Part model, mm, in its own coordinate system. Face numbers are marked on the shaded views. A direction names the side the tool comes from. Give positions to 0.01 mm unless a question says otherwise; leave off trailing zeros. Write each loop counter-clockwise with the first axis right and the second up, starting at its lowest first coordinate (ties: lowest second). Pieces come first, ordered by that corner, then holes. Notation, with made-up numbers: (12.5, 63) - (36.5, 63) arc R19 cw to (36.5, 81) - close; hole circle Ø2 at (40.5, 20.25). An arc over 180 degrees is marked (long way). Answer as a JSON object with one key per item and string values. Group by question number.
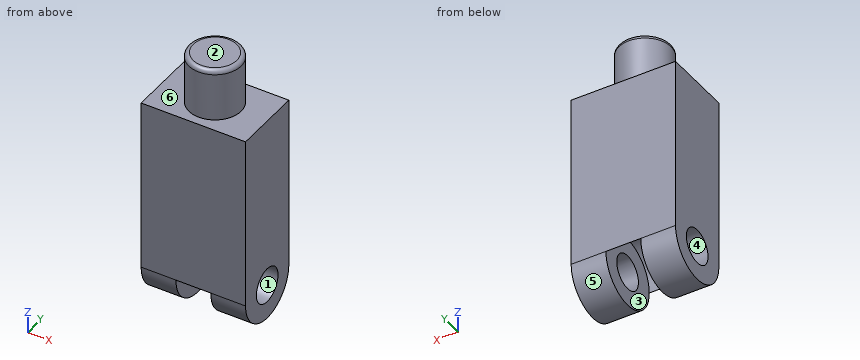
```python
from build123d import *

# Parameters (mm, degrees)
SKETCH_1_W               = 60
SKETCH_1_H               = 40
EXTRUDE_1_DEPTH          = 100
SKETCH_6_R               = 20
EXTRUDE_2_DEPTH          = 20
EXTRUDE_START            = -20
SKETCH_7_R               = 20
EXTRUDE_3_DEPTH          = 20
CUT_EXTRUDE_1_DEPTH      = 120.268604419
CUT_EXTRUDE_1_DEPTH_BACK = 120.268604419
SKETCH_8_R               = 10
SKETCH_9_R               = 20
CUT_EXTRUDE_2_DEPTH      = 20
SKETCH_10_R              = 15
EXTRUDE_4_DEPTH          = 30
FILLET_1_R               = 2.5


with BuildPart() as part:
    # 스케치1 → 보스-돌출1 (new body)
    with BuildSketch(Plane.XY):
        with Locations((20, 5)):
            Rectangle(SKETCH_1_W, SKETCH_1_H)
    extrude(amount=EXTRUDE_1_DEPTH)

    # 스케치6 → 보스-돌출2 (add)
    with BuildSketch(Plane(origin=(50, 0, 0), x_dir=(0, 0, -1), z_dir=(1, 0, 0))):
        with Locations((0, 5)):
            Circle(SKETCH_6_R)
    extrude(amount=-EXTRUDE_2_DEPTH)

    # 스케치7 → 보스-돌출3 (add)
    with BuildSketch(Plane.ZY.offset(10).offset(EXTRUDE_START)):
        with Locations((0, 5)):
            Circle(SKETCH_7_R)
    extrude(amount=EXTRUDE_3_DEPTH)

    # 스케치8 → 컷-돌출1 (cut, two sides: drawn at the far end of the back side and taken through both)
    with BuildSketch(Plane.ZY.offset(10).offset(-CUT_EXTRUDE_1_DEPTH_BACK)):
        with Locations((0, 5)):
            Circle(SKETCH_8_R)
    extrude(amount=CUT_EXTRUDE_1_DEPTH + CUT_EXTRUDE_1_DEPTH_BACK, mode=Mode.SUBTRACT)

    # 스케치9 → 컷-돌출2 (cut)
    with BuildSketch(Plane.ZY.offset(-30)):
        with Locations((0, 5)):
            Circle(SKETCH_9_R)
    extrude(amount=CUT_EXTRUDE_2_DEPTH, mode=Mode.SUBTRACT)

    # 스케치10 → 보스-돌출4 (add)
    with BuildSketch(Plane.XY.offset(100)):
        with Locations((20, 5)):
            Circle(SKETCH_10_R)
    extrude(amount=EXTRUDE_4_DEPTH)

    # 필렛1
    fillet_1_edges = [part.edges().sort_by_distance(p)[0] for p in [
        (5, 5, 130),
    ]]
    fillet(fillet_1_edges, radius=FILLET_1_R)


solid = part.part
```
1) Saw through at C-C (x = -6). List the corners of the cut face in (y, z).
2) Saw through at B-B (z = 8). List the corners of the cut face in (x, y), and give its area (3 significant figures).
3) Which spindle directions (+Z, -Z, +X, -X, +Y, -Y) get a long thin tool onto all of the face, cutting with end or side? Do the marked faces 5 and 6. Say none if no direction does.
4) Saw through at D-D (x = 20). List the corners of the cut face in (y, z), and give its area (3 significant figures).
5) Drop flat-ended pins along their axis: P1, Ø12, axis at y = 5, z = 0, coming from the -X side; P2, Ø1.5, axis at x = -1, y = 13.5, coming from the -Z side; P3, Ø10, axis at x = 36, y = 20.5, coming from the -Z side; P4, Ø6, axis at x = 24.5, y = -7, coming from the -Z side. Give the stop position or say it passes through.
6) Two-plate mould, pull along Z, no slides. Class the marked faces 1, 2, 3 and 4: +Z half, -Z half, draft (parallel to the pull), parting line (faces both ways), or undercut.
7) Saw through at A-A (y = 5). List the corners of the cut face in (x, z).
8) Drill centre lines: line 1 along Z through (x, y) = (4, 5); line 2 along Y through (x, z) = (42.5, 0); line 3 along Z through (x, y) = (7, 14). Where is each one in solid material? Low to high. Write a range as from..to.
Checks:
{
 "1": {"outline": "(-15, 0) arc R20 ccw to (25, 0) - (25, 100) - (-15, 100) - close; hole circle Ø20 at (5, 0)"},
 "2": {"outline": "(-10, -15) - (50, -15) - (50, -1) - (30, -1) - (30, -13.33) - (10, -13.33) - (10, -1) - (-10, -1) - close; (-10, 11) - (10, 11) - (10, 23.33) - (30, 23.33) - (30, 11) - (50, 11) - (50, 25) - (-10, 25) - close", "area": "1,190 mm2"},
 "3": {"face 5": "-Z, +X, -X", "face 6": "+Z"},
 "4": {"outline": "(-15, 0) arc R20 cw to (25, 0) - (25, 100) - (20, 100) - (20, 127.5) arc R2.5 ccw to (17.5, 130) - (-7.5, 130) arc R2.5 ccw to (-10, 127.5) - (-10, 100) - (-15, 100) - close", "area": "4,270 mm2"},
 "5": {"P1": "through", "P2": "z = -18.44", "P3": "z = -17.02", "P4": "z = 13.23"},
 "6": {"face 1": "undercut", "face 2": "+Z half", "face 3": "draft", "face 4": "undercut"},
 "7": {"outline": "(-10, -20) - (10, -20) - (10, -10) - (-10, -10) - close; (-10, 10) - (10, 10) - (10, 20) - (30, 20) - (30, 10) - (50, 10) - (50, 100) - (35, 100) - (35, 127.5) arc R2.5 ccw to (32.5, 130) - (7.5, 130) arc R2.5 ccw to (5, 127.5) - (5, 100) - (-10, 100) - close; (30, -20) - (50, -20) - (50, -10) - (30, -10) - close"},
 "8": {"line 1": "-20..-10, 10..100", "line 2": "-15..-5, 15..25", "line 3": "-17.86..-4.36, 4.36..100"}
}
